Source: CAD feature listing. Evaluate the final solid. Frame: model axes, mm. A direction names the side the tool comes from. Round coordinates to 2 decimals unless told otherwise and drop trailing zeros. Order: outer loops, then holes, each group sorted by start corner. A loop starts at its lowest first (then second) coordinate and runs counter-clockwise, first axis right, second up. Notation, with made-up numbers: M 71,40 L 77,40 A26 cw 77,64 Z; hole C 45,-30.5 d3. An arc over 180 degrees is marked long. Use one line per item in the form item = value. Start each with the question number.
Q1. Section B-B (x = 45). Return the cut outline in (y, z).
Q2. Section D-D (y = -24). Return the cut outline in (x, z), plus the area to 3 significant figures.
Q3. Contact query for flat-ended pins moving along their axis: pin 1 (1.5 mm diameter, centred on x = 26, y = -1.5, fed in from -Z); pin 2 (6 mm diameter, centred on x = -47, y = -0.5, fed in from +Z); pin 3 (9 mm diameter, centred on y = -8.5, z = 27, fed in from -X); pin 4 (6.5 mm diameter, centred on x = -86.5, z = -9.5, fed in from -Y). Output: stop coordinate, or through.
Q4. Section A-A (z = 0). Return the cut outline in (x, y) (3 decimals), plus the area to 3 significant figures.
Q5. Section C-C (y = -8). Return the cut outline in (x, z), plus the area to 3 significant figures.
Q6. Pull-direction query (Z, two-part tool) for faces 1 (the flat face through (98.225, 2, 0)), 2 (the cylindrical face through (-88.139, 2.465, 18.567)), 3 (the flat face through (-29, -10, 32.5)); classes: pulls with the +Z half, pulls with the -Z half, needs draft (parallel to the pull), parting line crosses it, or undercut.
Q7. Reachability of faces 4 (the flat face through (-76.25, -14, 0)), 5 (the flat face through (-13.75, -14, 0)), 6 (the flat face through (-45, -5, -21.25)), 7 (the flat face through (-54, -5, 27)) from +Z, -Z, +X, -X, +Y, -Y: full face, straight path, thin tool, end or side. Return the list, or none.
Q8. Material intervals for probe 1 along X at (y, z) = (2, 20) (3 decimals); probe 2 along X at (y, z) = (-7, 2); probe 3 along Z at (x, y) = (45, 2), sorted ascending.
from build123d import *

# Parameters (mm, degrees)
SKETCH2_W            = 196.45
SKETCH2_H            = 65
BOSS_EXTRUDE1_DEPTH  = 5
BOSS_EXTRUDE2_DEPTH  = 28
BOSS_EXTRUDE3_DEPTH  = 20
CUT_EXTRUDE9_START   = -33
CUT_EXTRUDE9_DEPTH   = 20
SKETCH4_R            = 26.99
CUT_EXTRUDE3_DEPTH   = 1.74
SKETCH3_4_R          = 19.2
CUT_EXTRUDE10_DEPTH  = 20
M3_CLEARANCE_HOLE1_D = 3.4


with BuildPart() as part:
    # Sketch2 → Boss-Extrude1 (new body)
    with BuildSketch(Plane(origin=(0, 0, 0), x_dir=(1, 0, 0), z_dir=(0, 1, 0))):
        Rectangle(SKETCH2_W, SKETCH2_H)
    extrude(amount=BOSS_EXTRUDE1_DEPTH)

    # Sketch3 → Boss-Extrude2 (add)
    with BuildSketch(Plane(origin=(0, 0, 0), x_dir=(1, 0, 0), z_dir=(0, 1, 0))):
        Polygon((-36, -32.5), (-36, -21.25), (-23.75, -21.25), (-23.75, 21.25), (-66.25, 21.25), (-66.25, -21.25), (-54, -21.25), (-54, -32.5), (-76.25, -32.5), (-76.25, 32.5), (-13.75, 32.5), (-13.75, -32.5), align=None)
    extrude(amount=-BOSS_EXTRUDE2_DEPTH)

    # Sketch12 → Boss-Extrude3 (add)
    with BuildSketch(Plane.XZ.offset(28)):
        Polygon((-36, 21.25), (-36, 32.5), (-54, 32.5), (-54, 21.25), (-66.25, 21.25), (-66.25, -21.25), (-23.75, -21.25), (-23.75, 21.25), align=None)
    extrude(amount=-BOSS_EXTRUDE3_DEPTH)

    # Sketch12<2> → Cut-Extrude9 (cut)
    with BuildSketch(Plane.XZ.offset(28).offset(CUT_EXTRUDE9_START)):
        Polygon((-36, 21.25), (-36, 32.5), (-54, 32.5), (-54, 21.25), (-66.25, 21.25), (-66.25, -21.25), (-23.75, -21.25), (-23.75, 21.25), align=None)
    extrude(amount=CUT_EXTRUDE9_DEPTH, mode=Mode.SUBTRACT)

    # Sketch4 → Cut-Extrude3 (cut)
    with BuildSketch(Plane(origin=(0, 5, 0), x_dir=(1, 0, 0), z_dir=(0, 1, 0))):
        with Locations((45, 0)):
            Circle(SKETCH4_R)
    extrude(amount=-CUT_EXTRUDE3_DEPTH, mode=Mode.SUBTRACT)

    # Sketch3<4> → Cut-Extrude10 (cut)
    with BuildSketch(Plane(origin=(0, 0, 0), x_dir=(1, 0, 0), z_dir=(0, 1, 0))):
        with Locations((45, 0)):
            Circle(SKETCH3_4_R)
    extrude(amount=CUT_EXTRUDE10_DEPTH, mode=Mode.SUBTRACT)

    # M3 Clearance Hole1 (through all)
    with Locations(Plane(origin=(0, 5, 0), x_dir=(1, 0, 0), z_dir=(0, 1, 0))):
        with Locations((-87.225, 20), (-87.225, 0), (-87.225, -20), (87.225, -20), (87.225, 0), (87.225, 20)):
            Hole(M3_CLEARANCE_HOLE1_D / 2)


solid = part.part
Results list:
q1.outline = M 0,-32.5 L 5,-32.5 L 5,-26.99 L 3.26,-26.99 L 3.26,-19.2 L 0,-19.2 Z; M 0,19.2 L 3.26,19.2 L 3.26,26.99 L 5,26.99 L 5,32.5 L 0,32.5 Z
q2.outline = M -76.25,-32.5 L -13.75,-32.5 L -13.75,32.5 L -76.25,32.5 Z
q2.area = 4,060 mm2
q3.pin_1 = through
q3.pin_2 = -21.25
q3.pin_3 = -76.25
q3.pin_4 = 0
q4.outline = M -98.225,0 L -88.925,0 L -88.925,5 L -98.225,5 Z; M -85.525,0 L -76.25,0 L -76.25,-28 L -13.75,-28 L -13.75,0 L 25.8,0 L 25.8,3.26 L 18.01,3.26 L 18.01,5 L -23.75,5 L -23.75,-15 L -66.25,-15 L -66.25,5 L -85.525,5 Z; M 64.2,0 L 85.525,0 L 85.525,5 L 71.99,5 L 71.99,3.26 L 64.2,3.26 Z; M 88.925,0 L 98.225,0 L 98.225,5 L 88.925,5 Z
q4.area = 1,630 mm2
q5.outline = M -76.25,-32.5 L -13.75,-32.5 L -13.75,32.5 L -36,32.5 L -36,21.25 L -23.75,21.25 L -23.75,-21.25 L -66.25,-21.25 L -66.25,21.25 L -54,21.25 L -54,32.5 L -76.25,32.5 Z
q5.area = 2,050 mm2
q6.face_1 = needs draft
q6.face_2 = undercut
q6.face_3 = pulls with the +Z half
q7.face_4 = +Z, -Z, -X, -Y
q7.face_5 = +Z, -Z, +X, -Y
q7.face_6 = +Y
q7.face_7 = +Z, +Y
q8.probe_1 = -98.225 to -88.925, -85.525 to -66.25, -23.75 to 85.525, 88.925 to 98.225
q8.probe_2 = -76.25 to -66.25, -23.75 to -13.75
q8.probe_3 = -32.5 to -19.2, 19.2 to 32.5
